The listing builds one solid part. Answer for the finished solid, in the listing's coordinates (mm). Face numbers are marked on the shaded views. A direction names the side the tool comes from. Round coordinates to 2 decimals unless told otherwise and drop trailing zeros. Write each loop counter-clockwise with the first axis right and the second up, starting at its lowest first coordinate (ties: lowest second). Pieces come first, ordered by that corner, then holes.
Item 1: Find section D-D on x = -107.5. Give the vertices of the cut face in (y, z).
Item 2: For a pull along X with two mould halves and no side action, classify the marked faces 3, 4, 5 and 6 as +X half, -X half, draft (parallel to the pull), parting line (faces both ways), or undercut.
Item 3: Find section C-C on y = -56. Give the vertices of the cut face in (x, z), then the cut area to 3 significant figures.
Item 4: A tool of negligible diameter and unlimited length cuts with its end or side. For the marked faces 1 and 2, from which of +Z, -Z, +X, -X, +Y, -Y can it reach the whole face along a straight path? Write none if from no direction.
Item 5: Find section B-B on z = 3.75. Give the vertices of the cut face in (x, y).
Item 6: Find section A-A on x = -83. Give the vertices of the cut face in (y, z).
Item 7: Find the intervals of material crossed by probe 1 along X at (y, z) = (-73, 0.75); probe 2 along Y at (x, z) = (-124.5, 2.75); probe 3 along Y at (x, z) = (-82.5, 4.5), in increasing order.
Item 8: Each of these flat-tipped pins is pushed along its axis until it touches: pin 1 (11 mm diameter, centred on x = -84.5, y = -68, fed in from -Z); pin 2 (1 mm diameter, centred on y = -61, z = 3, fed in from -X); pin 3 (3 mm diameter, centred on x = -33, z = 0.5, fed in from -Y); pin 4 (6.5 mm diameter, centred on x = -124.99, y = -71.6, fed in from -Z). Where does it stop, or does it pass through?
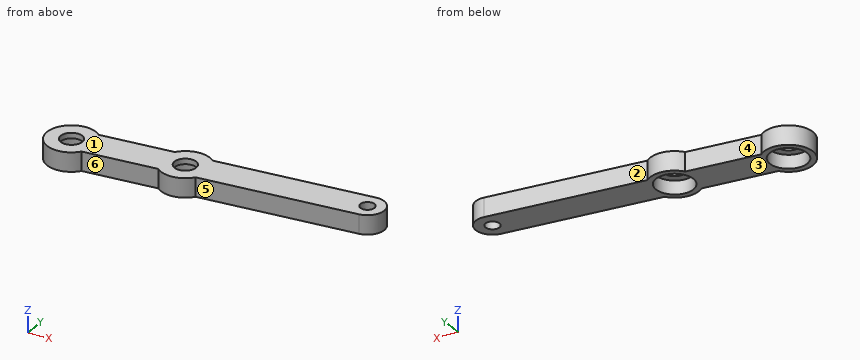
```python
from build123d import *

# Parameters (mm, degrees)
SKETCH1_R           = 2.6
SKETCH1_R_2         = 6.9
BOSS_EXTRUDE1_DEPTH = 5
SKETCH2_R           = 2.6
SKETCH2_R_2         = 4
BOSS_EXTRUDE2_DEPTH = 2


with BuildPart() as part:
    # Sketch1 → Boss-Extrude1 (new body)
    with BuildSketch(Plane.XY):
        with BuildLine():
            Line((-117.842377899, -77.068349263), (-91.221161774, -74.112086796))
            ThreePointArc((-91.221161774, -74.112086796), (-84.435913767, -76.1684327), (-78.267124508, -72.673552434))
            Line((-78.267124508, -72.673552434), (-21.451382857, -66.364214657))
            ThreePointArc((-21.451382857, -66.364214657), (-16.007105356, -59.559722092), (-22.811597922, -54.115444591))
            Line((-22.811597922, -54.115444591), (-79.542760834, -60.415389973))
            ThreePointArc((-79.542760834, -60.415389973), (-86.42258563, -58.278403776), (-92.665955577, -61.872709124))
            Line((-92.665955577, -61.872709124), (-119.079141177, -64.805869985))
            ThreePointArc((-119.079141177, -64.805869985), (-133.941604274, -72.498469269), (-117.842377899, -77.068349263))
        make_face()
        with Locations((-22.131490389, -60.239829624)):
            Circle(SKETCH1_R, mode=Mode.SUBTRACT)
        with Locations((-85.429249698, -67.223418238)):
            Circle(SKETCH1_R_2, mode=Mode.SUBTRACT)
        with Locations((-124.987033061, -71.595333402)):
            Circle(SKETCH1_R_2, mode=Mode.SUBTRACT)
    extrude(amount=BOSS_EXTRUDE1_DEPTH)

    # Sketch2 → Boss-Extrude2 (add)
    with BuildSketch(Plane.XY.offset(5)):
        with BuildLine():
            Line((-22.811597922, -54.115444591), (-79.542760834, -60.415389973))
            ThreePointArc((-79.542760834, -60.415389973), (-86.42258563, -58.278403776), (-92.665955577, -61.872709124))
            Line((-92.665955577, -61.872709124), (-119.079141177, -64.805869985))
            ThreePointArc((-119.079141177, -64.805869985), (-133.941604274, -72.498469269), (-117.842377899, -77.068349263))
            Line((-117.842377899, -77.068349263), (-91.221161774, -74.112086796))
            ThreePointArc((-91.221161774, -74.112086796), (-84.435913767, -76.1684327), (-78.267124508, -72.673552434))
            Line((-78.267124508, -72.673552434), (-21.451382857, -66.364214657))
            ThreePointArc((-21.451382857, -66.364214657), (-16.007105356, -59.559722092), (-22.811597922, -54.115444591))
        make_face()
        with Locations((-22.131490389, -60.239829624)):
            Circle(SKETCH2_R, mode=Mode.SUBTRACT)
        with Locations((-85.429249698, -67.223418238)):
            Circle(SKETCH2_R_2, mode=Mode.SUBTRACT)
        with Locations((-124.987033061, -71.595333402)):
            Circle(SKETCH2_R_2, mode=Mode.SUBTRACT)
    extrude(amount=BOSS_EXTRUDE2_DEPTH)


solid = part.part
```
Check values:
1. outline: (-75.92, 0) - (-63.52, 0) - (-63.52, 7) - (-75.92, 7) - close
2. face 3: draft
2. face 4: undercut
2. face 5: +X half
2. face 6: undercut
3. outline: (-39.78, 0) - (-17.66, 0) - (-17.66, 7) - (-39.78, 7) - close
3. area: 155 mm2
4. face 1: +Z, +X, -X, +Y, -Y
4. face 2: +Z, -Z, +Y
5. outline: (-119.08, -64.81) arc R9 ccw (long way) to (-117.84, -77.07) - (-91.22, -74.11) arc R9 ccw to (-78.27, -72.67) - (-21.45, -66.36) arc R6.16 ccw to (-22.81, -54.12) - (-79.54, -60.42) arc R9 ccw to (-92.67, -61.87) - close; hole circle Ø13.8 at (-124.99, -71.6); hole circle Ø13.8 at (-85.43, -67.22); hole circle Ø5.2 at (-22.13, -60.24)
6. outline: (-75.89, 0) - (-73.68, 0) - (-73.68, 5) - (-70.4, 5) - (-70.4, 7) - (-75.89, 7) - close; (-64.05, 5) - (-60.77, 5) - (-60.77, 0) - (-58.56, 0) - (-58.56, 7) - (-64.05, 7) - close
7. probe 1: x = -133.88 to -131.74, -118.23 to -89.2, -81.66 to -78.53
7. probe 2: y = -80.58 to -78.48, -64.71 to -62.61
7. probe 3: y = -75.73 to -73.47, -60.98 to -58.71
8. pin 1: stops at z = 5
8. pin 2: stops at x = -92.37
8. pin 3: stops at y = -67.81
8. pin 4: passes through
